from build123d import *

# Parameters (mm, degrees)
F0_W     = 100
F0_H     = 50
F1_DEPTH = 50
F2_T     = -10
F3_R     = 7.5
F4_DEPTH = 10.001
F5_W     = 6
F5_H     = 40
F6_DEPTH = 40
F7_SIZE  = 10
F8_SIZE  = 30


with BuildPart() as f1:
    # F0 (on Top) → F1 (new body)
    with BuildSketch(Plane.XY):
        Rectangle(F0_W, F0_H)
    extrude(amount=F1_DEPTH)

    # F2
    f2_openings = [f1.faces().sort_by_distance(p)[0] for p in [
        (50, 0, 25),
        (0, 0, 50),
        (0, -25, 25),
        (-50, 0, 25),
    ]]
    offset(amount=F2_T, openings=f2_openings)

    # F3 (on face) → F4 (cut, through all)
    with BuildSketch(Plane.XY.offset(10)):
        with Locations((-30, -5)):
            Circle(F3_R)
        with Locations((30, -5)):
            Circle(F3_R)
    extrude(amount=-F4_DEPTH, mode=Mode.SUBTRACT)

    # F5 (on face) → F6 (join, through all)
    with BuildSketch(Plane.XY.offset(10)):
        with Locations((0, -5)):
            Rectangle(F5_W, F5_H)
    extrude(amount=F6_DEPTH)

    # F7
    f7_edges = [f1.edges().sort_by_distance(p)[0] for p in [
        (50, 20, 50),
        (-50, 20, 50),
    ]]
    chamfer(f7_edges, length=F7_SIZE)

    # F8
    f8_edges = [f1.edges().sort_by_distance(p)[0] for p in [
        (0, -25, 50),
    ]]
    chamfer(f8_edges, length=F8_SIZE)


solid = f1.part
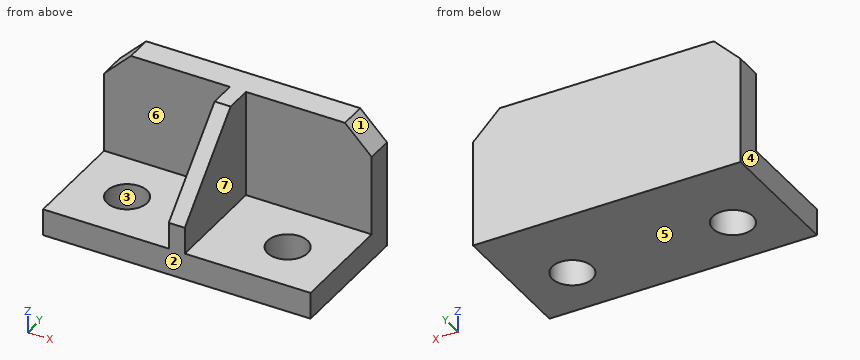
For this review, take the finished solid that the model builds, in its own axes (mm). Face numbers are marked on the shaded views. A direction names the side the tool comes from. Round coordinates to 2 decimals unless told otherwise and drop trailing zeros. Write each loop counter-clockwise with the first axis right and the second up, starting at its lowest first coordinate (ties: lowest second). Pieces come first, ordered by that corner, then holes. Notation, with made-up numbers: M 15,84 L 65,84 A17 cw 65,114 Z; hole C 75.25,19.5 d10. An arc over 180 degrees is marked long. Write item = value, one per line. Start each with the question number.
(1) We need section A-A (y = -5). Give the boundary of the cut face in (x, z), then the cut area to 3 significant figures.
(2) We need section C-C (z = 27.5). Give the boundary of the cut face in (x, y), then the cut area to 4 significant figures.
(3) Clearance check with flat-ended pins moving along their axes: pin 1 Ø1 at (x, y) = (11, 8) entering from -Z; pin 2 Ø20 at (x, y) = (-17, -7.5) entering from +Z; pin 3 Ø3 at (y, z) = (10, 41.5) entering from -X; pin 4 Ø20 at (x, z) = (22, 21.5) entering from -Y. State where each tip first meets the part, or that it passes through.
(4) We need section D-D (y = 21.5). Give the boundary of the cut face in (x, z).
(5) For the marked faces 5, 6 and 7, list the 3-axis set-ups (+Z, -Z, +X, -X, +Y, -Y) from which the entire face can be reached by the end or side of a thin tool; tool diameter is ignored.
(6) For line 1 along Y through (x, z) = (30, 5); line 2 along Z through (x, y) = (-14, -7); line 3 along Y through (x, z) = (-24, 4), list the stretches that pass through material, from the lowest coordinate up.
(7) The part is to be moulded in two halves that separate along X. For the marked faces 1, 2, 3 and 4, say which applies: +X half, -X half, draft (parallel to the pull), parting line (faces both ways), or undercut.
(8) We need section B-B (x = 30). Give the boundary of the cut face in (y, z).
Results found:
q1.outline = M -50,0 L -37.5,0 L -37.5,10 L -50,10 Z; M -22.5,0 L 22.5,0 L 22.5,10 L 3,10 L 3,40 L -3,40 L -3,10 L -22.5,10 Z; M 37.5,0 L 50,0 L 50,10 L 37.5,10 Z
q1.area = 880 mm²
q2.outline = M -50,15 L -3,15 L -3,-17.5 L 3,-17.5 L 3,15 L 50,15 L 50,25 L -50,25 Z
q2.area = 1,195 mm²
q3.pin_1 = 0
q3.pin_2 = 10
q3.pin_3 = -3
q3.pin_4 = 15
q4.outline = M -50,0 L 50,0 L 50,40 L 40,50 L -40,50 L -50,40 Z
q5.face_5 = -Z, +X, -X, +Y, -Y
q5.face_6 = +Z, -X, -Y
q5.face_7 = +Z, +X, -Y
q6.line_1 = -25 to -12.5, 2.5 to 25
q6.line_2 = 0 to 10
q6.line_3 = -25 to -9.5, -0.5 to 25
q7.face_1 = +X half
q7.face_2 = draft
q7.face_3 = undercut
q7.face_4 = -X half
q8.outline = M -25,0 L -12.5,0 L -12.5,10 L -25,10 Z; M 2.5,0 L 25,0 L 25,50 L 15,50 L 15,10 L 2.5,10 Z
